```python
from build123d import *

# Parameters (mm, degrees)
BOSS_EXTRUDE1_DEPTH = 2
SKETCH2_R           = 1
CUT_EXTRUDE1_DEPTH  = 3
FILLET2_R           = 3


with BuildPart() as part:
    # Sketch1 → Boss-Extrude1 (new body)
    with BuildSketch(Plane(origin=(0, 0, 0), x_dir=(1, 0, 0), z_dir=(0, 1, 0))):
        with BuildLine():
            Line((-30, 40), (30, 40))
            ThreePointArc((30, 40), (46.770509831, 36.041019662), (60, 25))
            Line((60, 25), (60, 0))
            ThreePointArc((60, 0), (46.770509831, 11.041019662), (30, 15))
            Line((30, 15), (-30, 15))
            ThreePointArc((-30, 15), (-46.770509831, 11.041019662), (-60, 0))
            Line((-60, 0), (-60, 25))
            ThreePointArc((-60, 25), (-46.770509831, 36.041019662), (-30, 40))
        make_face()
    extrude(amount=BOSS_EXTRUDE1_DEPTH)

    # Sketch2 → Cut-Extrude1 (cut)
    with BuildSketch(Plane(origin=(0, 2, 0), x_dir=(1, 0, 0), z_dir=(0, 1, 0))):
        with Locations(Location((56, 10, 0), (0, 0, 270))):
            Circle(SKETCH2_R)
        with Locations(Location((30, 36, 0), (0, 0, 270))):
            Circle(SKETCH2_R)
        with Locations(Location((-56, 10, 0), (0, 0, 90))):
            Circle(SKETCH2_R)
        with Locations(Location((-30, 36, 0), (0, 0, 90))):
            Circle(SKETCH2_R)
    extrude(amount=-CUT_EXTRUDE1_DEPTH, mode=Mode.SUBTRACT)

    # Fillet2
    fillet2_edges = [part.edges().sort_by_distance(p)[0] for p in [
        (-60, 1, 0),
        (-60, 1, -25),
        (60, 1, -25),
        (60, 1, 0),
    ]]
    fillet(fillet2_edges, radius=FILLET2_R)


solid = part.part
```
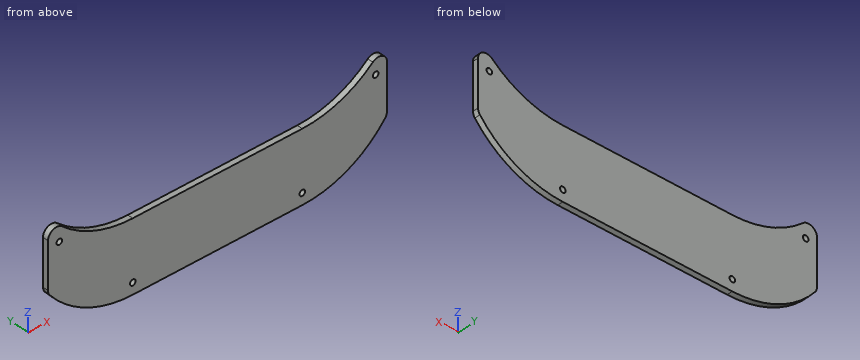
Build history of the part. All positions in model axes, mm. Round coordinates to 2 decimals unless told otherwise and drop trailing zeros. Order: outer loops, then holes, each group sorted by start corner. A loop starts at its lowest first (then second) coordinate and runs counter-clockwise, first axis right, second up. Notation, with made-up numbers: (2, 11.25) -> (41, 11.25) arc R23 ccw to (41, 30.25) -> close; hole circle Ø10 at (-28.75, 25.25). An arc over 180 degrees is marked (long way). Answer in a Markdown table with one row per item.
1) Band-saw the part on B-B on x = 41. Give the cut face in (y, z), and give its area (3 significant figures).
Values:
| item | result |
|---|---|
| outline | (0, -38.35) -> (2, -38.35) -> (2, -13.35) -> (0, -13.35) -> close |
| area | 50.0 mm2 |
2) Pin check, flat tip, straight feed: P1, Ø0.6, axis at x = 11, y = 0.5, coming from the +Z side. Stop position of the tip, or through.
Values:
| item | result |
|---|---|
| P1 | z = -15 |
3) Wall check: L1, parallel to Z at x = -30, y = 0.8; L2, parallel to X at y = 1.1, z = -36; L3, parallel to Z at x = 9, y = 1.35. Give the ranges that are in metal, low to high.
Values:
| item | result |
|---|---|
| L1 | -40 to -37, -35 to -15 |
| L2 | -46.85 to -31, -29 to 29, 31 to 46.85 |
| L3 | -40 to -15 |
4) Band-saw the part on A-A on y = 0.3. Give the cut face in (x, z), and give its area (3 significant figures).
Values:
| item | result |
|---|---|
| outline | (-60, -23.98) arc R3 ccw to (-59.35, -25.84) arc R37.5 ccw to (-30, -40) -> (30, -40) arc R37.5 ccw to (59.35, -25.84) arc R3 ccw to (60, -23.98) -> (60, -7.69) arc R3 ccw to (55, -5.45) arc R37.5 cw to (30, -15) -> (-30, -15) arc R37.5 cw to (-55, -5.45) arc R3 ccw to (-60, -7.69) -> close; hole circle Ø2 at (-56, -10); hole circle Ø2 at (-30, -36); hole circle Ø2 at (30, -36); hole circle Ø2 at (56, -10) |
| area | 2,960 mm2 |
